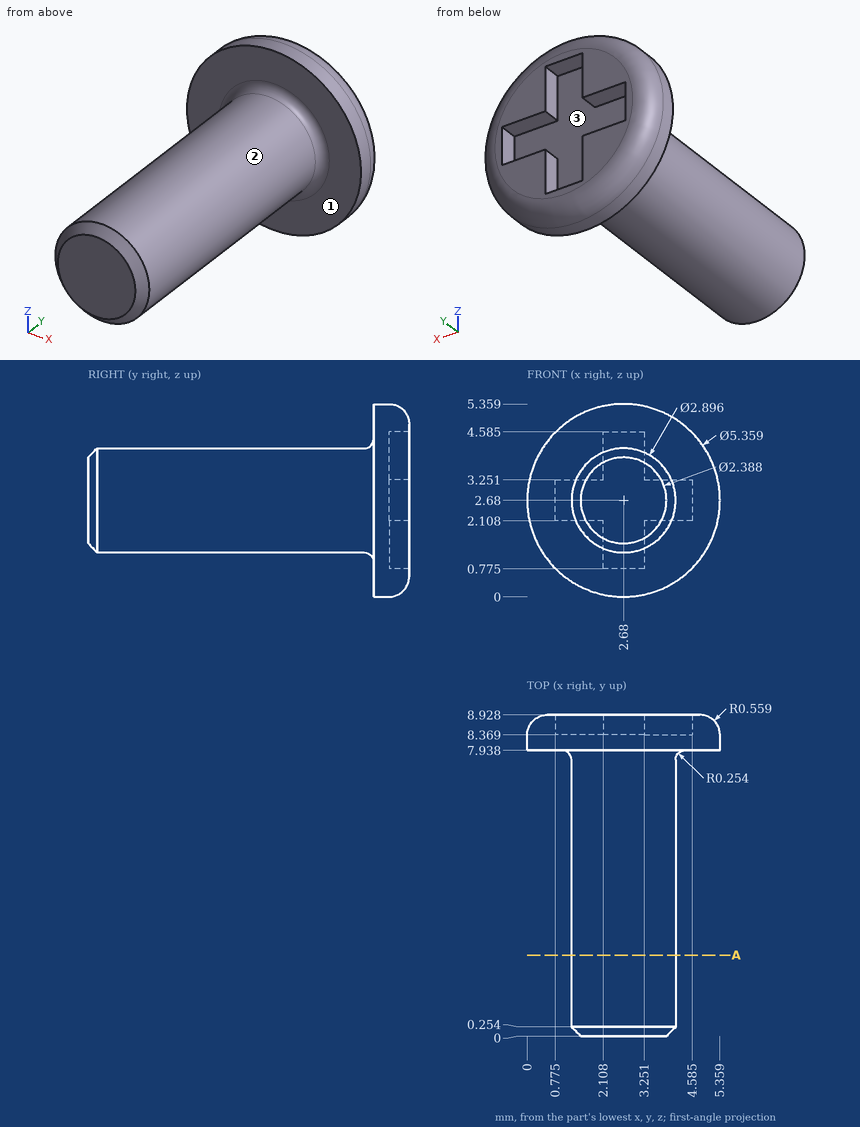
Job drawing, mm, ordinate dimensions from the low corner. One solid piece. Give positions to 0.01 mm unless a question says otherwise; leave off trailing zeros. Loops run counter-clockwise (first coordinate to the right, second up) from the corner with the lowest first, then second, coordinate; pieces in that order, holes last. Notation, with made-up numbers: (65.25, 22) -> (74.25, 22) arc R25 ccw to (74.25, 53) -> close; hole circle Ø6 at (49.5, 42). An arc over 180 degrees is marked (long way). Write each question's results on one line, items separated by ' | '.
(1) Probe line 1 along Y through (x, z) = (3.7, 3.2); line 2 along X through (y, z) = (6.75, 2.6) (1 decimal); line 3 along Y through (x, z) = (2.3, 0.7). List the from-to ranges inside material, lowest first.
Geometry results:
line 1: y = 0 to 8.37 | line 2: x = 1.2 to 4.1 | line 3: y = 7.94 to 8.93
(2) Flat gauge pins, fed straight in: pin 1 Ø0.6 at (x, y) = (1.5, 8.5) entering from +Z (1 decimal); pin 2 Ø0.6 at (y, z) = (9, 4) entering from -X (1 decimal); pin 3 Ø0.6 at (x, y) = (3.5, 9) entering from +Z (1 decimal). Where does each tip first touch, or does it go through?
Geometry results:
pin 1: stops at z = 5.2 | pin 2: stops at x = 0.4 | pin 3: stops at z = 5.1
(3) Cut at A-A on y = 2.25. List the corners of the cut face in (x, z) (1 decimal).
Geometry results:
outline: circle Ø2.9 at (2.7, 2.7)
(4) Pull direction Z, two halves, no side cores. Call the marked faces 1, 2 and 3: released by +Z, released by -Z, zero draft, split by the parting line, or undercut.
Geometry results:
face 1: zero draft | face 2: split by the parting line | face 3: undercut
